Read the model definition and answer for the solid it produces. Units are mm, in the model's axes. Face numbers are marked on the shaded views. A direction names the side the tool comes from. Coordinates: 2 decimals unless noted, no trailing zeros. Loops run counter-clockwise (first coordinate to the right, second up) from the corner with the lowest first, then second, coordinate; pieces in that order, holes last. Notation, with made-up numbers: (-17, 63.25) -> (22, 63.25) arc R24 cw to (22, 75.25) -> close; hole circle Ø1 at (23.5, -16.75). An arc over 180 degrees is marked (long way). Answer as a JSON object with one key per item and string values. Group by question number.
Q1. Straight lines are drawn through the part: line 1 along Y through (x, z) = (-0.7, -0.65); line 2 along Y through (x, z) = (-0.5, -1.9); line 3 along Z through (x, y) = (-0.05, 7). For each, find the intervals that lie inside material, in ascending order. Write a range as [from, to].
Q2. Determine the mould class of the marked faces 1, 2 and 3 for opening direction Z: released by +Z, released by -Z, zero draft, split by the parting line, or undercut.
Q3. The part is cut by section A-A on x = 0. Write down the section's boundary in (y, z).
Q4. Each of these flat-tipped pins is pushed along its axis until it touches: P1, Ø3, axis at y = 7, z = -1, coming from the +X side; P2, Ø1, axis at x = 1.5, y = 2.5, coming from the -Z side; P3, Ø3, axis at x = -2, y = 2, coming from the -Z side. Where does it stop, or does it pass through?
Q5. For the marked faces 4, 5 and 6, determine the directions among +Z, -Z, +X, -X, +Y, -Y from which every point of the face is accessible in a straight line to the end or side of a thin tool.
Q6. The part is cut by section B-B on y = 2. Write down the section's boundary in (x, z), and give its area (3 significant figures).
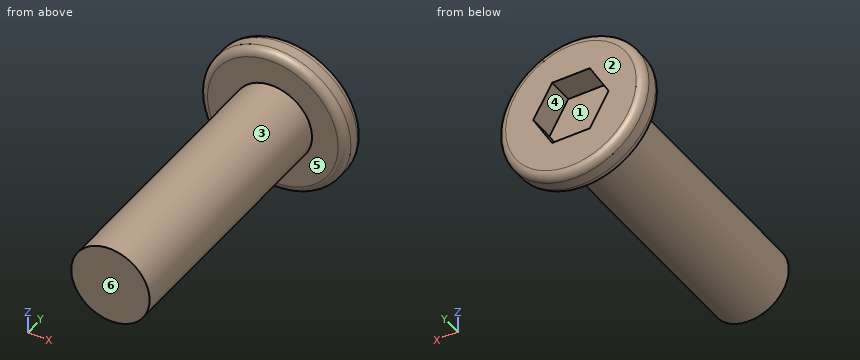
from build123d import *

# Parameters (mm, degrees)
SKETCH_1_R          = 1.5
EXTRUDE_1_DEPTH     = 10
SKETCH_2_R          = 2.8
EXTRUDE_2_DEPTH     = 1
CUT_EXTRUDE_1_DEPTH = 1
FILLET_1_R          = 0.3


with BuildPart() as part:
    # 草图1 → 凸台-拉伸1 (new body)
    with BuildSketch(Plane(origin=(0, 0, 0), x_dir=(1, 0, 0), z_dir=(0, 1, 0))):
        with Locations(Location((0, 0, 0), (0, 0, 270))):
            Circle(SKETCH_1_R)
    extrude(amount=EXTRUDE_1_DEPTH)

    # 草图2 → 凸台-拉伸2 (add)
    with BuildSketch(Plane(origin=(0, 10, 0), x_dir=(1, 0, 0), z_dir=(0, 1, 0))):
        with Locations(Location((0, 0, 0), (0, 0, 270))):
            Circle(SKETCH_2_R)
    extrude(amount=EXTRUDE_2_DEPTH)

    # 草图3 → 切除-拉伸1 (cut)
    with BuildSketch(Plane(origin=(0, 11, 0), x_dir=(1, 0, 0), z_dir=(0, 1, 0))):
        Polygon((-1.443375673, 0), (-0.721687836, -1.25), (0.721687836, -1.25), (1.443375673, 0), (0.721687836, 1.25), (-0.721687836, 1.25), align=None)
    extrude(amount=-CUT_EXTRUDE_1_DEPTH, mode=Mode.SUBTRACT)

    # 圆角1
    fillet_1_edges = [part.edges().sort_by_distance(p)[0] for p in [
        (0, 10, -2.8),
        (0, 11, -2.8),
    ]]
    fillet(fillet_1_edges, radius=FILLET_1_R)


solid = part.part
Final values:
{
 "1": {"line 1": "y = [0, 10]", "line 2": "y = [10, 11]", "line 3": "z = [-1.5, 1.5]"},
 "2": {"face 1": "undercut", "face 2": "zero draft", "face 3": "split by the parting line"},
 "3": {"outline": "(0, -1.5) -> (10, -1.5) -> (10, -2.5) arc R0.3 ccw to (10.3, -2.8) -> (10.7, -2.8) arc R0.3 ccw to (11, -2.5) -> (11, -1.25) -> (10, -1.25) -> (10, 1.25) -> (11, 1.25) -> (11, 2.5) arc R0.3 ccw to (10.7, 2.8) -> (10.3, 2.8) arc R0.3 ccw to (10, 2.5) -> (10, 1.5) -> (0, 1.5) -> close"},
 "4": {"P1": "stops at x = 1.5", "P2": "stops at z = -1.12", "P3": "stops at z = -1.41"},
 "5": {"face 4": "+Y", "face 5": "-Y", "face 6": "+Z, -Z, +X, -X, -Y"},
 "6": {"outline": "circle Ø3 at (0, 0)", "area": "7.07 mm2"}
}
